Read the model definition and answer for the solid it produces. Units are mm, in the model's axes. A direction names the side the tool comes from. Coordinates: 2 decimals unless noted, no trailing zeros. Order: outer loops, then holes, each group sorted by start corner. A loop starts at its lowest first (then second) coordinate and runs counter-clockwise, first axis right, second up.
```python
from build123d import *

# Parameters (mm, degrees)
SKETCH_1_R          = 1.05
EXTRUDE_1_DEPTH     = 55
SKETCH_2_W          = 51
SKETCH_2_H          = 5
CUT_EXTRUDE_1_DEPTH = 15
SKETCH_3_R          = 1.5
CUT_EXTRUDE_2_DEPTH = 15
SKETCH_4_W          = 20
SKETCH_4_H          = 21.363917142
CUT_EXTRUDE_3_DEPTH = 12


with BuildPart() as part:
    # 草图1 → 凸台-拉伸1 (new body)
    with BuildSketch(Plane.XY):
        Polygon((-11, 10), (-20, 10), (-40, -10), (-11, -10), (-11, -7), (11, -7), (11, -10), (40, -10), (20, 10), (11, 10), (11, 7.5), (-11, 7.5), align=None)
        with Locations((-30.525046877, -6.313107933)):
            Circle(SKETCH_1_R, mode=Mode.SUBTRACT)
        with Locations((-20.062564905, -2.241948818)):
            Circle(SKETCH_1_R, mode=Mode.SUBTRACT)
        with Locations((30.525046877, -6.313107933)):
            Circle(SKETCH_1_R, mode=Mode.SUBTRACT)
        with Locations((20.062564905, -2.241948818)):
            Circle(SKETCH_1_R, mode=Mode.SUBTRACT)
    extrude(amount=EXTRUDE_1_DEPTH)

    # 草图2 → 切除-拉伸1 (cut)
    with BuildSketch(Plane.XZ.offset(10)):
        Polygon((-40, 45), (-25.5, 45), (-11, 45), (-11, 50), (-25.5, 50), (-40, 50), align=None)
        with Locations((14.5, 47.5)):
            Rectangle(SKETCH_2_W, SKETCH_2_H)
        Polygon((-11, 40), (-25.5, 40), (-40, 40), (-40, 35), (-25.5, 35), (-11, 35), align=None)
        with Locations((14.5, 37.5)):
            Rectangle(SKETCH_2_W, SKETCH_2_H)
        Polygon((-25.5, 30), (-40, 30), (-40, 25), (-25.5, 25), (-11, 25), (-11, 30), align=None)
        with Locations((14.5, 27.5)):
            Rectangle(SKETCH_2_W, SKETCH_2_H)
        Polygon((-25.5, 20), (-40, 20), (-40, 15), (-25.5, 15), (-11, 15), (-11, 20), align=None)
        with Locations((14.5, 17.5)):
            Rectangle(SKETCH_2_W, SKETCH_2_H)
        Polygon((-25.5, 10), (-40, 10), (-40, 5), (-25.5, 5), (-11, 5), (-11, 10), align=None)
        with Locations((14.5, 7.5)):
            Rectangle(SKETCH_2_W, SKETCH_2_H)
    extrude(amount=-CUT_EXTRUDE_1_DEPTH, mode=Mode.SUBTRACT)

    # 草图3 → 切除-拉伸2 (cut)
    with BuildSketch(Plane(origin=(0, 7.5, 0), x_dir=(1, 0, 0), z_dir=(0, 1, 0))):
        with BuildLine():
            ThreePointArc((1.5, -20.5), (1.060660172, -19.439339828), (0, -19))
            Line((0, -19), (0, -22))
            ThreePointArc((0, -22), (1.060660172, -21.560660172), (1.5, -20.5))
        make_face()
        with BuildLine():
            Line((0, -22), (0, -19))
            ThreePointArc((0, -19), (-1.5, -20.5), (0, -22))
        make_face()
        with BuildLine():
            ThreePointArc((1.7, -27.5), (1.202081528, -26.297918472), (0, -25.8))
            Line((0, -25.8), (0, -29.2))
            ThreePointArc((0, -29.2), (1.202081528, -28.702081528), (1.7, -27.5))
        make_face()
        with BuildLine():
            Line((0, -29.2), (0, -25.8))
            ThreePointArc((0, -25.8), (-1.7, -27.5), (0, -29.2))
        make_face()
        with Locations(Location((-7, -27.5, 0), (0, 0, 270))):
            Circle(SKETCH_3_R)
        with Locations(Location((7, -27.5, 0), (0, 0, 270))):
            Circle(SKETCH_3_R)
        with BuildLine():
            ThreePointArc((1.5, -34.5), (1.060660172, -33.439339828), (0, -33))
            Line((0, -33), (0, -36))
            ThreePointArc((0, -36), (1.060660172, -35.560660172), (1.5, -34.5))
        make_face()
        with BuildLine():
            Line((0, -36), (0, -33))
            ThreePointArc((0, -33), (-1.5, -34.5), (0, -36))
        make_face()
    extrude(amount=-CUT_EXTRUDE_2_DEPTH, mode=Mode.SUBTRACT)

    # 草图4 → 切除-拉伸3 (cut)
    with BuildSketch(Plane.XZ.offset(7)):
        with Locations((0, 27.5)):
            Rectangle(SKETCH_4_W, SKETCH_4_H)
    extrude(amount=-CUT_EXTRUDE_3_DEPTH, mode=Mode.SUBTRACT)


solid = part.part
```
1) Which of the six approach directions +Z, -Z, +X, -X, +Y, -Y give full straight-line access (tool end or side, diameter ignored) to faces 5 (the flat face through (22, -3, 30)), 6 (the flat face through (0, -7, 52)), 7 (the flat face through (25, -10, 42))?
A:
face 5: +X, -X, -Y
face 6: +Z, -Z, -Y
face 7: +Z, -Z, +X, -X, -Y
2) A cutting plane is placed at C-C, the plane x = -7. Determine the outline of the cut face in (y, z), and give its area (3 significant figures).
A:
outline: (-7, 0) - (7.5, 0) - (7.5, 26) - (5, 26) - (5, 15) - (-7, 15) - (-7, 10) - (5, 10) - (5, 5) - (-7, 5) - close; (-7, 40) - (5, 40) - (5, 29) - (7.5, 29) - (7.5, 55) - (-7, 55) - (-7, 50) - (5, 50) - (5, 45) - (-7, 45) - close
area: 370 mm2
3) A cutting plane is placed at D-D, the plane x = 13.5. Determine the outline of the cut face in (y, z).
A:
outline: (-10, 0) - (10, 0) - (10, 55) - (-10, 55) - (-10, 50) - (5, 50) - (5, 45) - (-10, 45) - (-10, 40) - (5, 40) - (5, 35) - (-10, 35) - (-10, 30) - (5, 30) - (5, 25) - (-10, 25) - (-10, 20) - (5, 20) - (5, 15) - (-10, 15) - (-10, 10) - (5, 10) - (5, 5) - (-10, 5) - close
4) Determine the mould class of faces 1 (the flat face through (-28, 2, 21)), 2 (the flat face through (-1, -3, 45)), 3 (the flat face through (-10, -1, 22)), 4 (the flat face through (-10, -1, 32)) for opening direction X: pulls with the +X half, pulls with the -X half, needs draft (parallel to the pull), parting line crosses it, or undercut.
A:
face 1: pulls with the -X half
face 2: needs draft
face 3: undercut
face 4: undercut
5) A cutting plane is placed at B-B, the plane y = 6.5. Determine the outline of the cut face in (x, z), and give its area (3 significant figures).
A:
outline: (-23.5, 0) - (23.5, 0) - (23.5, 55) - (-23.5, 55) - close; hole circle Ø3 at (-7, 27.5); hole circle Ø3.4 at (0, 27.5); hole circle Ø3 at (0, 20.5); hole circle Ø3 at (0, 34.5); hole circle Ø3 at (7, 27.5)
area: 2,550 mm2
6) Flat-ended cylindrical pins translate along their axes: pin 1 Ø3.5 at (y, z) = (-9, 41.5) entering from -X; pin 2 Ø0.5 at (x, z) = (10.5, 33) entering from -Y; pin 3 Ø1.5 at (x, z) = (29, 42.5) entering from +Y. Find the tip coordinate at first contact, or state that the pin passes through.
A:
pin 1: stops at x = -40
pin 2: stops at y = -7
pin 3: stops at y = 1.75
7) A cutting plane is placed at A-A, the plane x = 33. Determine the outline of the cut face in (y, z), and give its area (3 significant figures).
A:
outline: (-10, 0) - (-3, 0) - (-3, 5) - (-10, 5) - close; (-10, 10) - (-3, 10) - (-3, 15) - (-10, 15) - close; (-10, 20) - (-3, 20) - (-3, 25) - (-10, 25) - close; (-10, 30) - (-3, 30) - (-3, 35) - (-10, 35) - close; (-10, 40) - (-3, 40) - (-3, 45) - (-10, 45) - close; (-10, 50) - (-3, 50) - (-3, 55) - (-10, 55) - close
area: 210 mm2
8) Straight lines are drawn through the part: line 1 (Z direction, x = 32, y = -6.5); line 2 (Z direction, x = 5, y = -2.75); line 3 (Y direction, x = 18.5, z = 37.5). For each, find the intervals that lie inside material, in ascending order.
A:
line 1: z = 0 to 5, 10 to 15, 20 to 25, 30 to 35, 40 to 45, 50 to 55
line 2: z = 0 to 5, 10 to 15, 40 to 45, 50 to 55
line 3: y = 5 to 10
